Here's how the part is built. I have some questions about the finished solid (model axes, mm). A direction names the side the tool comes from. Coordinates: 2 decimals unless noted, no trailing zeros. Write each loop counter-clockwise with the first axis right and the second up, starting at its lowest first coordinate (ties: lowest second). Pieces come first, ordered by that corner, then holes.
Item 1: We'd pull the mould along X, two halves only. Please class faces 1 (the face through (-20, 3, 0)), 2 (the face through (-27, 3, -10.1)), 3 (the face through (28.7, 3, -17.9)), 4 (the face through (0, 3, 19.5)): +X half, -X half, draft (parallel to the pull), parting line (faces both ways), or undercut.
Item 2: If we section it at A-A (x = -14): Please give me the cut outline in (y, z), then the cut area to 3 significant figures.
Item 3: For faces 5 (the face through (-27, 3, 10.099)), 6 (the face through (-27, 3, 21)), 7 (the face through (0, 3, -19.5)), 8 (the face through (34, 3, -15)), 9 (the face through (-34, 3, -15)), which set-ups out of +Z, -Z, +X, -X, +Y, -Y let a thin tool reach every point of the face, with its end or its side?
Item 4: If I drill on line 1 (X direction, y = 2.5, z = -13); line 2 (X direction, y = 1.6, z = 11); line 3 (X direction, y = 0.85, z = -14), over which ranges is the centre line in solid material (lowest first)?
Item 5: If we section it at B-B (x = 23.5): Please give me the cut outline in (y, z), then the cut area to 3 significant figures.
Item 6: If we section it at C-C (z = -12): Please give me the cut outline in (x, y).
Item 7: I'm going to push flat-ended pins straight in: pin 1 Ø3 at (y, z) = (2.5, -16.5) entering from -X; pin 2 Ø1.8 at (y, z) = (3, -1) entering from -X; pin 3 Ø3 at (y, z) = (3.5, -1.5) entering from +X. Where does each tip first touch, or does it pass through?
from build123d import *

# Parameters (mm, degrees)
SKETCH1_R           = 2.55
BOSS_EXTRUDE1_DEPTH = 6
FILLET1_R           = 0.74
FILLET2_R           = 0.5


with BuildPart() as part:
    # Sketch1 → Boss-Extrude1 (new body)
    with BuildSketch(Plane(origin=(0, 0, 0), x_dir=(1, 0, 0), z_dir=(0, 1, 0))):
        with BuildLine():
            Line((-19.26, -19.5), (19.26, -19.5))
            ThreePointArc((19.26, -19.5), (19.783259018, -19.716740982), (20, -20.24))
            Line((20, -20.24), (20, -20.26))
            ThreePointArc((20, -20.26), (20.216740982, -20.783259018), (20.74, -21))
            Line((20.74, -21), (34.2, -21))
            Line((34.2, -21), (34.2, -10.099009877))
            Line((34.2, -10.099009877), (20, -10.099009877))
            Line((20, -10.099009877), (20, 10.1))
            Line((20, 10.1), (34, 10.1))
            Line((34, 10.1), (34, 21))
            Line((34, 21), (20.74, 21))
            ThreePointArc((20.74, 21), (20.216740982, 20.783259018), (20, 20.26))
            Line((20, 20.26), (20, 20.24))
            ThreePointArc((20, 20.24), (19.783259018, 19.716740982), (19.26, 19.5))
            Line((19.26, 19.5), (-19.26, 19.5))
            ThreePointArc((-19.26, 19.5), (-19.783259018, 19.716740982), (-20, 20.24))
            Line((-20, 20.24), (-20, 20.26))
            ThreePointArc((-20, 20.26), (-20.216740982, 20.783259018), (-20.74, 21))
            Line((-20.74, 21), (-34, 21))
            Line((-34, 21), (-34, 10.1))
            Line((-34, 10.1), (-20, 10.1))
            Line((-20, 10.1), (-20, -10.099009877))
            Line((-20, -10.099009877), (-34.2, -10.099009877))
            Line((-34.2, -10.099009877), (-34.2, -21))
            Line((-34.2, -21), (-20.74, -21))
            ThreePointArc((-20.74, -21), (-20.216740982, -20.783259018), (-20, -20.26))
            Line((-20, -20.26), (-20, -20.24))
            ThreePointArc((-20, -20.24), (-19.783259018, -19.716740982), (-19.26, -19.5))
        make_face()
        with Locations(Location((-14, 13, 0), (0, 0, 270))):
            Circle(SKETCH1_R, mode=Mode.SUBTRACT)
        with Locations(Location((14, 13, 0), (0, 0, 90))):
            Circle(SKETCH1_R, mode=Mode.SUBTRACT)
        with Locations(Location((14, -13, 0), (0, 0, 270))):
            Circle(SKETCH1_R, mode=Mode.SUBTRACT)
        with Locations(Location((-14, -13, 0), (0, 0, 90))):
            Circle(SKETCH1_R, mode=Mode.SUBTRACT)
        with Locations(Location((27, 16, 0), (0, 0, 270))):
            Circle(SKETCH1_R, mode=Mode.SUBTRACT)
        with Locations(Location((27, -16, 0), (0, 0, 90))):
            Circle(SKETCH1_R, mode=Mode.SUBTRACT)
        with Locations(Location((-27, -16, 0), (0, 0, 270))):
            Circle(SKETCH1_R, mode=Mode.SUBTRACT)
        with Locations(Location((-27, 16, 0), (0, 0, 90))):
            Circle(SKETCH1_R, mode=Mode.SUBTRACT)
    extrude(amount=BOSS_EXTRUDE1_DEPTH)

    # Fillet1
    fillet1_edges = [part.edges().sort_by_distance(p)[0] for p in [
        (34.2, 3, 21),
        (-34.2, 3, 21),
        (-34, 3, -21),
        (34, 3, -21),
    ]]
    fillet(fillet1_edges, radius=FILLET1_R)

    # Fillet2
    fillet2_edges = [part.edges().sort_by_distance(p)[0] for p in [
        (27.1, 6, 10.099009877),
        (-27, 6, -10.1),
        (-27.1, 6, 10.099009877),
        (27, 6, -10.1),
    ]]
    fillet(fillet2_edges, radius=FILLET2_R)


solid = part.part
Answer list:
1. face 1: -X half
1. face 2: draft
1. face 3: undercut
1. face 4: undercut
2. outline: (0, -19.5) - (6, -19.5) - (6, -15.55) - (0, -15.55) - close; (0, -10.45) - (6, -10.45) - (6, 10.45) - (0, 10.45) - close; (0, 15.55) - (6, 15.55) - (6, 19.5) - (0, 19.5) - close
2. area: 173 mm2
3. face 5: -X, +Y, -Y
3. face 6: +Z, +X, -X, +Y, -Y
3. face 7: -Z, +Y, -Y
3. face 8: -Z, +X, +Y, -Y
3. face 9: -Z, -X, +Y, -Y
4. line 1: x = -34 to -16.55, -11.45 to 11.45, 16.55 to 34
4. line 2: x = -34.2 to -15.58, -12.42 to 12.42, 15.58 to 34.2
4. line 3: x = -34 to -28.58, -25.42 to -16.35, -11.65 to 11.65, 16.35 to 25.42, 28.58 to 34
5. outline: (0, -21) - (6, -21) - (6, -10.6) arc R0.5 ccw to (5.5, -10.1) - (0, -10.1) - close; (0, 10.1) - (5.5, 10.1) arc R0.5 ccw to (6, 10.6) - (6, 21) - (0, 21) - close
5. area: 131 mm2
6. outline: (-34, 0) - (-16.35, 0) - (-16.35, 6) - (-34, 6) - close; (-11.65, 0) - (11.65, 0) - (11.65, 6) - (-11.65, 6) - close; (16.35, 0) - (34, 0) - (34, 6) - (16.35, 6) - close
7. pin 1: stops at x = -34
7. pin 2: stops at x = -20
7. pin 3: stops at x = 20
